Autodesk Inventor part; units mm, degrees
ref_plane "YZ Plane" through (0, 0, 0) normal (1, 0, 0) x (0, 1, 0)
ref_plane "XZ Plane" through (0, 0, 0) normal (0, 1, 0) x (-1, 0, 0)
ref_plane "XY Plane" through (0, 0, 0) normal (0, 0, 1) x (1, 0, 0)
sketch "Szkic3" plane through (0, 0, 0) normal (0, 1, 0) x (-1, 0, 0)
  line L0 (0, 0) -> (-20, 0)
  line L1 (-20, 0) -> (-20, -20)
  line L2 (-20, -20) -> (0, -20)
  line L3 (0, -20) -> (0, 0)
  dimension "d6" = 20
  dimension "d7" = 20
extrude "Wyciągnięcie proste3" add sketch "Szkic3" along normal blind 5
sketch "Szkic4" plane through (0, 0, 0) normal (0, -1, 0) x (1, 0, 0)
  line L0 (0, 0) -> (20, 0)
  line L1 (20, 0) -> (20, -20)
  line L2 (0, 0) -> (20, -20)
  line L3 (20, -20) -> (20, 0)
  line L4 (20, 0) -> (0, 0)
extrude "Wyciągnięcie proste4" cut sketch "Szkic4" against normal blind 5
sketch "Szkic5" plane through (0, 5, 0) normal (0, 1, 0) x (1, 0, 0)
  line L0 (20, 20) -> (0, 20)
  line L1 (0, 20) -> (25.3553, 45.3553)
  line L2 (0, 20) -> (35.8579, 20) construction
  line L3 (0, 0) -> (20, 20)
  line L4 (0, 0) -> (35.3553, 35.3553)
  line L5 (0, 0) -> (50, 0) construction
  line L6 (10.8927, 30.8927) -> (33.735, 53.735)
  line L7 (10.8927, 30.8927) -> (43.1966, 30.8927) construction
  line L8 (35.3553, 35.3553) -> (25.3553, 45.3553)
  dimension "d12" = 45
  dimension "d13" = 50
  dimension "d14" = 45
  dimension "d15" = 45
extrude "Wyciągnięcie proste5" add sketch "Szkic5" against normal blind 5
properties part number "Helenowiak_podpora"
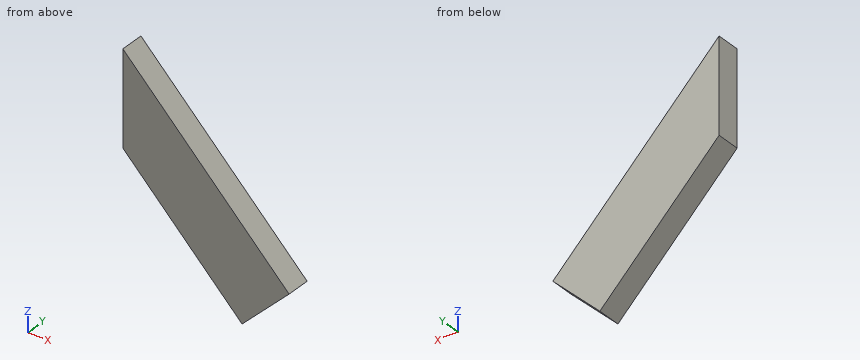
The listing builds one solid part. Answer for the finished solid, in the listing's coordinates (mm). Give positions to 0.01 mm unless a question says otherwise; leave off trailing zeros. Order: outer loops, then holes, each group sorted by start corner. A loop starts at its lowest first (then second) coordinate and runs counter-clockwise, first axis right, second up.
1) Consider line 1 along X through (y, z) = (0.85, -8); line 2 along X through (y, z) = (3.9, -7.5); line 3 along Z through (x, y) = (18.5, 3.05). Determine where each line is inside the solid, lowest interval first.
Reported:
line 1: x = 0 to 8
line 2: x = 0 to 7.5
line 3: z = -38.5 to -18.5
2) Find section B-B on y = 2.05. Write down the section's boundary in (x, z).
Reported:
outline: (0, -20) - (25.36, -45.36) - (35.36, -35.36) - (0, 0) - close
3) Find section A-A on z = -4.5. Write down the section's boundary in (x, y).
Reported:
outline: (0, 0) - (4.5, 0) - (4.5, 5) - (0, 5) - close
4) Given P1, Ø2, axis at y = 1, z = -32, coming from the +X side; P2, Ø1, axis at x = 10.5, z = -14, coming from the -Y side; P3, Ø1.5, axis at x = 8.5, y = 1, coming from the -Z side, each flat-ended and moving along its own axis, determine where each tip first touches the part or whether it passes through.
Reported:
P1: stops at x = 33
P2: stops at y = 0
P3: stops at z = -29.25
